Work out the finished part from the listing and answer in its coordinate system (mm). A direction names the side the tool comes from. Give positions to 0.01 mm unless a question says otherwise; leave off trailing zeros. Order: outer loops, then holes, each group sorted by start corner. A loop starts at its lowest first (then second) coordinate and runs counter-clockwise, first axis right, second up. Notation, with made-up numbers: (80, 21.25) -> (119, 21.25) arc R22 cw to (119, 33.25) -> close; hole circle Ø7 at (24, 15.25). An arc over 180 degrees is marked (long way). Use a Markdown table: item, result. Add a question column.
```python
from build123d import *

# Parameters (mm, degrees)
F0_W      = 90
F0_H      = 60
F1_DEPTH  = 4
F3_DEPTH  = 90
F4_W      = 2.2
F4_H      = 2.2
F4_W_2    = 2.5
F4_H_2    = 2.3
F5_DEPTH  = 90
F4_H_3    = 0.7
F6_DEPTH  = 90
F7_W      = 25
F7_H      = 2.2
F8_DEPTH  = 2.2
F9_W      = 26
F9_H      = 2.5
F10_DEPTH = 1.7
F11_SIZE  = 0.5


with BuildPart() as f1:
    # F0 (on Top) → F1 (new body)
    with BuildSketch(Plane.XY):
        Rectangle(F0_W, F0_H)
    extrude(amount=F1_DEPTH)

    # F2 (on face) → F3 (join, through all)
    with BuildSketch(Plane.YZ.offset(45)):
        Polygon((22, 102.5777145975), (5.1942216862, 4), (25, 4), (25, 102.5777145975), align=None)
        Polygon((-30, 10), (-30, 4), (5.1942216862, 4), align=None)
    extrude(amount=-F3_DEPTH)

    # F4 (on face) → F5 (cut, through all)
    with BuildSketch(Plane.YZ.offset(45)):
        with Locations((-28.9, 1.1)):
            Rectangle(F4_W, F4_H)
        Polygon((-27.8, 2.2), (-27.8, 0), (-25, 0), (-25, 5), (-27.8, 5), align=None)
        with Locations((26.25, 2.85)):
            Rectangle(F4_W_2, F4_H_2)
    extrude(amount=-F5_DEPTH, mode=Mode.SUBTRACT)

    # F4 (on face) → F6 (join, through all)
    with BuildSketch(Plane.YZ.offset(45)):
        with Locations((28.75, 4.35)):
            Rectangle(F4_W_2, F4_H_3)
    extrude(amount=-F6_DEPTH)

    # F7 (on face) → F8 (join, through all)
    with BuildSketch(Plane(origin=(0, 0, 2.2), x_dir=(1, 0, 0), z_dir=(0, 0, -1))):
        with Locations((0, 28.9)):
            Rectangle(F7_W, F7_H)
    extrude(amount=F8_DEPTH)

    # F9 (on face) → F10 (cut, through all)
    with BuildSketch(Plane.XY.offset(1.7)):
        with Locations((0, 26.25)):
            Rectangle(F9_W, F9_H)
    extrude(amount=-F10_DEPTH, mode=Mode.SUBTRACT)

    # F11
    f11_edges = [f1.edges().sort_by_distance(p)[0] for p in [
        (0, 30, 4.7),
        (0, 27.5, 4.7),
        (-13, 26.25, 1.7),
        (13, 26.25, 1.7),
    ]]
    chamfer(f11_edges, length=F11_SIZE)


solid = f1.part
```
1) The part is cut by section B-B, the plane z = 45.5. Determine the outline of the cut face in (x, y).
2) Flat-ended cylindrical pins translate along their axes: pin 1 (0.7 mm diameter, centred on y = -29, z = 1, fed in from -X); pin 2 (1.8 mm diameter, centred on x = -24, y = -29, fed in from -Z); pin 3 (1.2 mm diameter, centred on x = -22.5, y = 28.5, fed in from +Z). Find the tip coordinate at first contact, or state that the pin passes through.
3) The part is cut by section A-A, the plane x = -15.5. Determine the outline of the cut face in (y, z).
4) Which of the six approach directions +Z, -Z, +X, -X, +Y, -Y give full straight-line access (tool end or side, diameter ignored) to faces 1 (the flat face through (0.63, -12.16, 6.96)), 2 (the flat face through (-1, 3, 0)), 3 (the flat face through (1, -26, 5))?
5) Determine the mould class of faces 4 (the flat face through (1, 27.5, 3)), 5 (the flat face through (1, -30, 6)), 6 (the flat face through (-45, 15, 33)), 7 (the flat face through (1, 30, 2)) for opening direction Y: released by +Y, released by -Y, zero draft, split by the parting line, or undercut.
6) Straight lines are drawn through the part: line 1 (Z direction, x = -35.5, y = -4); line 2 (Y direction, x = -40, z = 21); line 3 (Z direction, x = 33, y = -11). For each, find the intervals that lie inside material, in ascending order.
7) The part is cut by section C-C, the plane y = -3. Determine the outline of the cut face in (x, z).
A:
| question | item | result |
|---|---|---|
| 1 | outline | (-45, 12.27) -> (45, 12.27) -> (45, 25) -> (-45, 25) -> close |
| 2 | pin 1 | x = -12.5 |
| 2 | pin 2 | z = 2.2 |
| 2 | pin 3 | z = 4.7 |
| 3 | outline | (-30, 2.2) -> (-27.8, 2.2) -> (-27.8, 5) -> (-25, 5) -> (-25, 0) -> (30, 0) -> (30, 4.2) -> (29.5, 4.7) -> (28, 4.7) -> (27.5, 4.2) -> (27.5, 1.7) -> (25, 1.7) -> (25, 102.58) -> (22, 102.58) -> (5.19, 4) -> (-30, 10) -> close |
| 4 | face 1 | +Z, +X, -X |
| 4 | face 2 | -Z, +X, -X, +Y, -Y |
| 4 | face 3 | -Z, +X, -X |
| 5 | face 4 | undercut |
| 5 | face 5 | released by -Y |
| 5 | face 6 | zero draft |
| 5 | face 7 | released by +Y |
| 6 | line 1 | 0 to 5.57 |
| 6 | line 2 | 8.09 to 25 |
| 6 | line 3 | 0 to 6.76 |
| 7 | outline | (-45, 0) -> (45, 0) -> (45, 5.4) -> (-45, 5.4) -> close |
